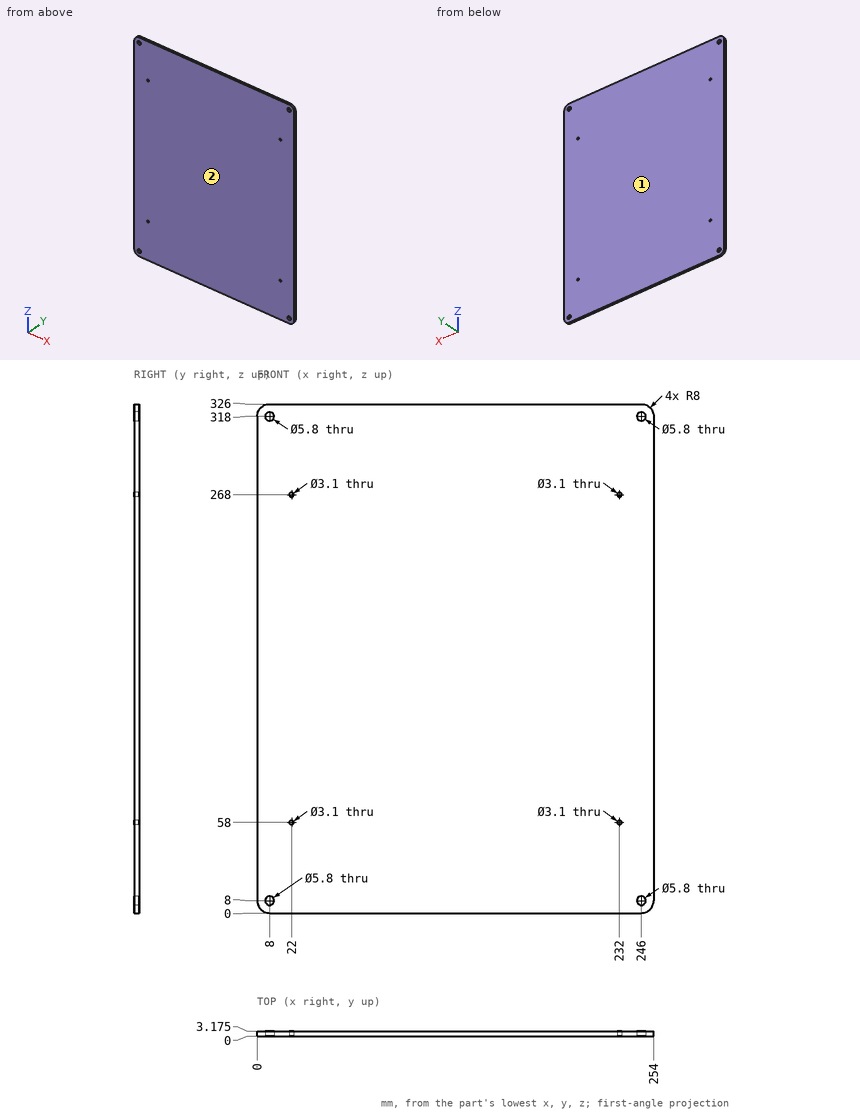
Design review of the part shown in the three views and the two pictorial views. Dimensions are in mm from the part's minimum x, y and z. Round coordinates to 2 decimals unless told otherwise and drop trailing zeros.
1) The part is to be moulded in two halves that separate along Y. For the marked faces 1 and 2, say which applies: pulls with the +Y half, pulls with the -Y half, needs draft (parallel to the pull), parting line crosses it, or undercut.
Values follow:
face 1: pulls with the +Y half
face 2: pulls with the -Y half
2) Clearance check with a flat-ended pin moving along its axis: P1, Ø3.5, axis at x = 232, z = 58, coming from the +Y side (3 decimals). State where the tip first meets the part, or that it passes through.
Values follow:
P1: stops at y = 3.175
3) Wall thickness on line 1 along Z through (x, y) = (232, 2.2); line 2 along X through (y, z) = (0.7, 318); line 3 along X through (y, z) = (1.15, 58): over which ranges is each line inside the solid? List them lowest first.
Values follow:
line 1: z = 0 to 56.45, 59.55 to 266.45, 269.55 to 326
line 2: x = 0 to 5.1, 10.9 to 243.1, 248.9 to 254
line 3: x = 0 to 20.45, 23.55 to 230.45, 233.55 to 254
